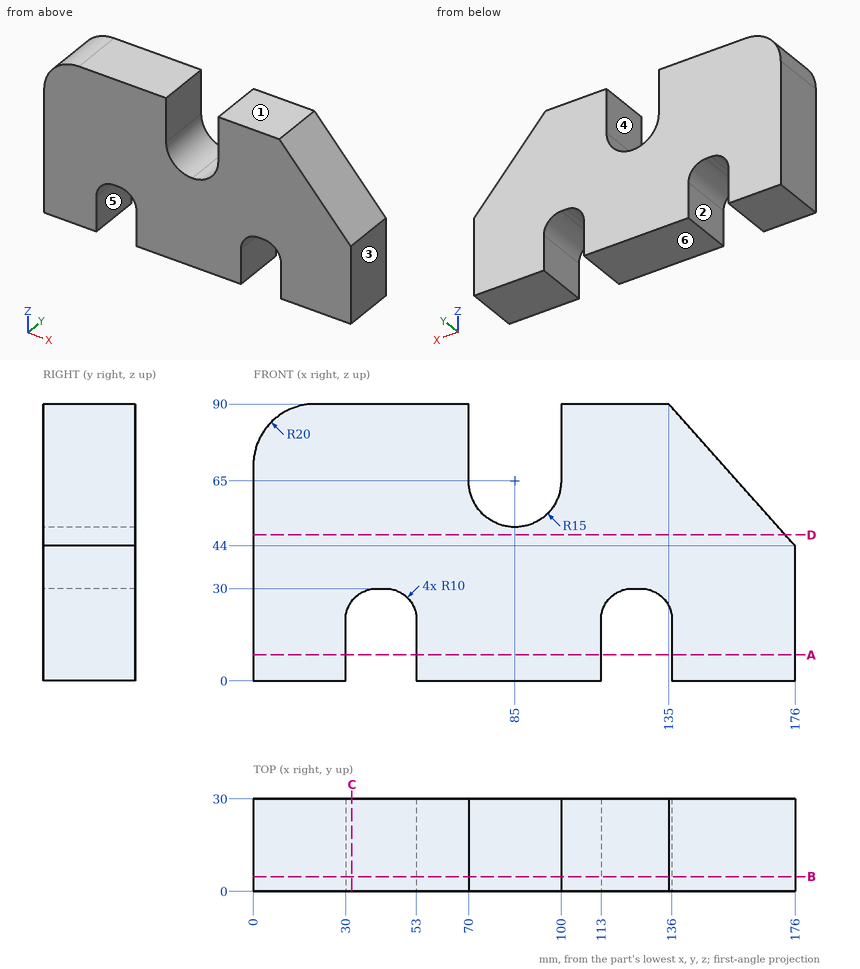
Geometry: see drawing. Coordinates: mm, zero at the bounding-box minimum. A direction names the side the tool comes from. Coordinates: 2 decimals unless noted, no trailing zeros. Write each loop counter-clockwise with the first axis right and the second up, starting at its lowest first coordinate (ties: lowest second). Pieces come first, ordered by that corner, then holes.
1) Mould query, pull axis X, two halves, no side actions, for the marked faces 1, 2 and 3. Classes: pulls with the +X half, pulls with the -X half, needs draft (parallel to the pull), parting line crosses it, or undercut.
2) Section D-D on z = 47.5. Output: boundary loops of the cut face in (x, y).
3) Set-up query: the marked faces 4, 5 and 6. Return all of +Z, -Z, +X, -X, +Y, -Y with unobstructed straight access to the full face (end or side cutting, diameter ignored); none if empty.
4) Section A-A on z = 8.5. Output: boundary loops of the cut face in (x, y).
5) Section B-B on y = 4.75. Output: boundary loops of the cut face in (x, z), and give its area (3 significant figures).
6) Pin query (flat end, axial travel): pin 1 Ø4 at (x, y) = (127, 5.5) entering from -Z; pin 2 Ø0.9 at (x, y) = (124.5, 11.5) entering from -Z; pin 3 Ø3 at (y, z) = (13, 77.5) entering from -X. Return the tip coordinate at first contact, or that it passes through.
7) Section C-C on x = 32. Output: boundary loops of the cut face in (y, z).
8) Material intervals for line 1 along X through (y, z) = (6.5, 15.5); line 2 along X through (y, z) = (28.25, 70); line 3 along X through (y, z) = (2, 86), sorted ascending.
Check result:
1. face 1: needs draft
1. face 2: undercut
1. face 3: pulls with the +X half
2. outline: (0, 0) - (172.88, 0) - (172.88, 30) - (0, 30) - close
3. face 4: +Z, +Y, -Y
3. face 5: -Z, +Y, -Y
3. face 6: -Z, +X, -X, +Y, -Y
4. outline: (0, 0) - (30, 0) - (30, 30) - (0, 30) - close; (53, 0) - (113, 0) - (113, 30) - (53, 30) - close; (136, 0) - (176, 0) - (176, 30) - (136, 30) - close
5. outline: (0, 0) - (30, 0) - (30, 20) arc R10 cw to (40, 30) - (43, 30) arc R10 cw to (53, 20) - (53, 0) - (113, 0) - (113, 20) arc R10 cw to (123, 30) - (126, 30) arc R10 cw to (136, 20) - (136, 0) - (176, 0) - (176, 44) - (135, 90) - (100, 90) - (100, 65) arc R15 cw to (85, 50) arc R15 cw to (70, 65) - (70, 90) - (20, 90) arc R20 ccw to (0, 70) - close
5. area: 12,400 mm2
6. pin 1: stops at z = 29.54
6. pin 2: stops at z = 30
6. pin 3: stops at x = 0.92
7. outline: (0, 26) - (30, 26) - (30, 90) - (0, 90) - close
8. line 1: x = 0 to 30, 53 to 113, 136 to 176
8. line 2: x = 0 to 70, 100 to 152.83
8. line 3: x = 8 to 70, 100 to 138.57
